Model file for the job. Use its own axes, mm. Coordinates: 2 decimals unless noted, no trailing zeros. Order: outer loops, then holes, each group sorted by start corner. A loop starts at its lowest first (then second) coordinate and runs counter-clockwise, first axis right, second up.
Autodesk Inventor part; units mm, degrees
ref_plane "YZ Plane" through (0, 0, 0) normal (1, 0, 0) x (0, 1, 0)
ref_plane "XZ Plane" through (0, 0, 0) normal (0, 1, 0) x (-1, 0, 0)
ref_plane "XY Plane" through (0, 0, 0) normal (0, 0, 1) x (1, 0, 0)
sketch "Sketch1" plane through (0, 0, 0) normal (0, 1, 0) x (-1, 0, 0)
  line L0 (0, 0) -> (25.4, 0)
  line L1 (25.4, 0) -> (25.4, -25.4)
  line L2 (25.4, -25.4) -> (0, -25.4)
  line L3 (0, -25.4) -> (0, 0)
  line L4 (23.8125, -23.8125) -> (23.8125, -1.5875)
  line L5 (23.8125, -1.5875) -> (1.5875, -1.5875)
  line L6 (1.5875, -1.5875) -> (1.5875, -23.8125)
  line L7 (1.5875, -23.8125) -> (23.8125, -23.8125)
  dimension "d0" = 25.4
  dimension "d1" = 25.4
  dimension "d2" = 1.5875
extrude "Extrusion1" add sketch "Sketch1" against normal blind 1219.2
properties part number "Square Tube" material "Aluminum 6061"
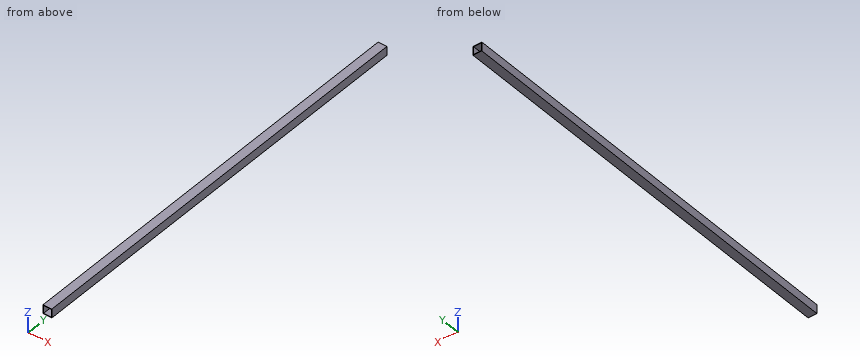
Q1. Probe line 1 (X direction, y = -743.5, z = -18). List the from-to ranges inside material, lowest first.
Established:
line 1: x = -25.4 to -23.81, -1.59 to 0
Q2. Cut at C-C, the plane y = -478. List the corners of the cut face in (x, z).
Established:
outline: (-25.4, -25.4) - (0, -25.4) - (0, 0) - (-25.4, 0) - close; hole (-23.81, -23.81) - (-1.59, -23.81) - (-1.59, -1.59) - (-23.81, -1.59) - close
Q3. Cut at A-A, the plane x = -6.75. List the corners of the cut face in (y, z), plus the area to 3 significant figures.
Established:
outline: (-1219.2, -25.4) - (0, -25.4) - (0, -23.81) - (-1219.2, -23.81) - close; (-1219.2, -1.59) - (0, -1.59) - (0, 0) - (-1219.2, 0) - close
area: 3,870 mm2
Q4. Cut at B-B, the plane z = -9.25. List the corners of the cut face in (x, y), plus the area to 3 significant figures.
Established:
outline: (-25.4, -1219.2) - (-23.81, -1219.2) - (-23.81, 0) - (-25.4, 0) - close; (-1.59, -1219.2) - (0, -1219.2) - (0, 0) - (-1.59, 0) - close
area: 3,870 mm2
